Build history of the part. All positions in model axes, mm. Face numbers are marked on the shaded views. Round coordinates to 2 decimals unless told otherwise and drop trailing zeros. Loops run counter-clockwise (first coordinate to the right, second up) from the corner with the lowest first, then second, coordinate; pieces in that order, holes last. Notation, with made-up numbers: (19, 22) - (32, 22) arc R28 ccw to (32, 45) - close; hole circle Ø8 at (15, 63.25). An arc over 180 degrees is marked (long way). Put each result on its own line as item: value. Start each with the question number.
from build123d import *

# Parameters (mm, degrees)
ESQUISSE1_W                  = 440
ESQUISSE1_H                  = 440
ESQUISSE1_W_2                = 380
ESQUISSE1_H_2                = 380
BOSS_EXTRU_1_DEPTH           = 40
ENL_V_MAT_EXTRU_1_DEPTH      = 390
ENL_V_MAT_EXTRU_1_DEPTH_BACK = 10
ESQUISSE2_W                  = 400
ESQUISSE2_H                  = 10
ESQUISSE3_W                  = 42
ESQUISSE3_H                  = 42
BOSS_EXTRU_2_DEPTH           = 80
ESQUISSE5_R                  = 2
BOSS_EXTRU_3_DEPTH           = 15
ESQUISSE7_R                  = 4
ENL_V_MAT_EXTRU_2_DEPTH      = 20
ESQUISSE8_W                  = 30
ESQUISSE8_H                  = 30
BOSS_EXTRU_4_DEPTH           = 41


with BuildPart() as part:
    # Esquisse1 → Boss.-Extru.1 (new body)
    with BuildSketch(Plane.XY):
        Rectangle(ESQUISSE1_W, ESQUISSE1_H)
        Rectangle(ESQUISSE1_W_2, ESQUISSE1_H_2, mode=Mode.SUBTRACT)
    extrude(amount=BOSS_EXTRU_1_DEPTH)

    # Esquisse2 → Enlèv. mat.-Extru.1 (cut, two sides: drawn at the far end of the back side and taken through both)
    with BuildSketch(Plane(origin=(0, -190, 0), x_dir=(1, 0, 0), z_dir=(0, 1, 0)).offset(-ENL_V_MAT_EXTRU_1_DEPTH_BACK)):
        with Locations((0, -20)):
            Rectangle(ESQUISSE2_W, ESQUISSE2_H)
    extrude(amount=ENL_V_MAT_EXTRU_1_DEPTH + ENL_V_MAT_EXTRU_1_DEPTH_BACK, mode=Mode.SUBTRACT)

    # Esquisse3 → Boss.-Extru.2 (add)
    with BuildSketch(Plane(origin=(0, 0, 0), x_dir=(-1, 0, 0), z_dir=(0, 0, -1))):
        with Locations((-199, 199)):
            Rectangle(ESQUISSE3_W, ESQUISSE3_H)
        with Locations((199, 199)):
            Rectangle(ESQUISSE3_W, ESQUISSE3_H)
    extrude(amount=BOSS_EXTRU_2_DEPTH)

    # Esquisse5 → Boss.-Extru.3 (add)
    with BuildSketch(Plane(origin=(0, 0, -80), x_dir=(-1, 0, 0), z_dir=(0, 0, -1))):
        with Locations((-210.505010618, 210.505010618)):
            Circle(ESQUISSE5_R)
        with Locations((-189.505010618, 189.505010618)):
            Circle(ESQUISSE5_R)
        with Locations(Location((215.288490097, 215.288490097, 0), (0, 0, 180))):
            Circle(ESQUISSE5_R)
        with Locations(Location((194.288490097, 194.288490097, 0), (0, 0, 180))):
            Circle(ESQUISSE5_R)
    extrude(amount=BOSS_EXTRU_3_DEPTH)

    # Esquisse7 → Enlèv. mat.-Extru.2 (cut)
    with BuildSketch(Plane.XZ.offset(-178)):
        with Locations(Location((199, -60.5, 0), (0, 0, 270))):
            Circle(ESQUISSE7_R)
        with Locations(Location((-199, -60.5, 0), (0, 0, 270))):
            Circle(ESQUISSE7_R)
    extrude(amount=-ENL_V_MAT_EXTRU_2_DEPTH, mode=Mode.SUBTRACT)

    # Esquisse8 → Boss.-Extru.4 (add)
    with BuildSketch(Plane(origin=(0, 0, 0), x_dir=(-1, 0, 0), z_dir=(0, 0, -1))):
        with Locations((-205, -205)):
            Rectangle(ESQUISSE8_W, ESQUISSE8_H)
        with Locations((205, -205)):
            Rectangle(ESQUISSE8_W, ESQUISSE8_H)
    extrude(amount=BOSS_EXTRU_4_DEPTH)


solid = part.part
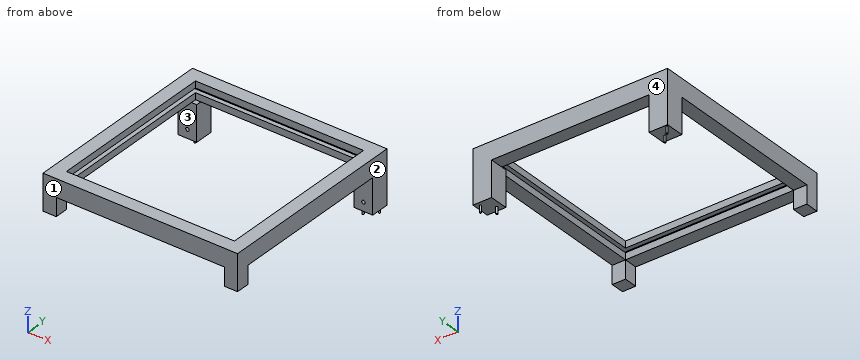
Item 1: Slice it at A-A (x = -113). Give the cut face in (y, z), plus the area to 3 significant figures.
Item 2: Drop flat-ended pins along their axis: pin 1 Ø9 at (x, y) = (211, -203.5) entering from -Z; pin 2 Ø15 at (x, y) = (-205, -23.5) entering from -Z. Give the stop position or say it passes through.
Item 3: Drill centre lines: probe 1 along X at (y, z) = (-61, 19.5); probe 2 along X at (y, z) = (189.75, -60.5); probe 3 along X at (y, z) = (192, -3.5). Where is each one in solid material? Low to high. Write a range as [from, to].
Item 4: Slice it at B-B (z = -23). Give the cut face in (x, y).
Item 5: Two-plate mould, pull along Y, no slides. Class the marked faces 1, 2, 3 and 4: pulls with the +Y half, pulls with the -Y half, needs draft (parallel to the pull), parting line crosses it, or undercut.
Item 6: Slice it at C-C (z = 8). Give the cut face in (x, y).
Computed values:
1. outline: (-220, 0) - (-190, 0) - (-190, 15) - (-200, 15) - (-200, 25) - (-190, 25) - (-190, 40) - (-220, 40) - close; (190, 0) - (220, 0) - (220, 40) - (190, 40) - (190, 25) - (200, 25) - (200, 15) - (190, 15) - close
1. area: 2,200 mm^2
2. pin 1: stops at z = -41
2. pin 2: stops at z = 0
3. probe 1: x = [-220, -200], [200, 220]
3. probe 2: x = [-220, -203], [-195, -178], [178, 195], [203, 220]
3. probe 3: x = [-220, -178], [178, 220]
4. outline: (-220, -220) - (-190, -220) - (-190, -190) - (-220, -190) - close; (-220, 178) - (-178, 178) - (-178, 220) - (-220, 220) - close; (178, 178) - (220, 178) - (220, 220) - (178, 220) - close; (190, -220) - (220, -220) - (220, -190) - (190, -190) - close
5. face 1: pulls with the -Y half
5. face 2: needs draft
5. face 3: undercut
5. face 4: pulls with the +Y half
6. outline: (-220, -220) - (220, -220) - (220, 220) - (-220, 220) - close; hole (-190, -190) - (190, -190) - (190, 190) - (-190, 190) - close
